Can you work these out from the model? Positions are in its coordinate system, mm. A direction names the side the tool comes from. Round coordinates to 2 decimals unless told otherwise and drop trailing zeros. Loops run counter-clockwise (first coordinate to the right, second up) from the corner with the lowest first, then second, coordinate; pieces in that order, holes last.
from build123d import *

# Parameters (mm, degrees)
BOSS_EXTRUDE1_DEPTH = 150
SKETCH2_R           = 35
SKETCH2_R_2         = 32.5
BOSS_EXTRUDE2_DEPTH = 14
SKETCH3_R           = 9
BOSS_EXTRUDE3_DEPTH = 8
SKETCH5_R           = 3.4
CUT_EXTRUDE1_DEPTH  = 14
CUT_EXTRUDE4_DEPTH  = 154
CUT_EXTRUDE6_START  = -4
CUT_EXTRUDE6_DEPTH  = 4
CUT_EXTRUDE7_START  = -4
CUT_EXTRUDE7_DEPTH  = 4
SKETCH13_R          = 3.4
CUT_EXTRUDE8_DEPTH  = 10
CIRPATTERN1_COUNT   = 3


with BuildPart() as part:
    # Sketch1 → Boss-Extrude1 (new body)
    with BuildSketch(Plane.YZ):
        Polygon((-60, -45), (-60, 45), (60, 45), (60, -45), (56, -45), (56, 41), (-56, 41), (-56, -45), align=None)
    extrude(amount=BOSS_EXTRUDE1_DEPTH)

    # Sketch2 → Boss-Extrude2 (add)
    with BuildSketch(Plane(origin=(0, 60, 0), x_dir=(-1, 0, 0), z_dir=(0, 1, 0))):
        with Locations(Location((-105.539679059, 0.129309752, 0), (0, 0, 270))):
            Circle(SKETCH2_R)
        with Locations(Location((-105.539679059, 0.129309752, 0), (0, 0, 90))):
            Circle(SKETCH2_R_2, mode=Mode.SUBTRACT)
    extrude(amount=BOSS_EXTRUDE2_DEPTH)

    # Sketch3 → Boss-Extrude3 (add)
    with BuildSketch(Plane(origin=(0, 60, 0), x_dir=(-1, 0, 0), z_dir=(0, 1, 0))):
        with Locations(Location((-105.539679059, 0.129309752, 0), (0, 0, 270))):
            Circle(SKETCH3_R)
        with BuildLine():
            Line((-109.989679059, -5.274161354), (-101.089679059, -5.274161354))
            ThreePointArc((-101.089679059, -5.274161354), (-105.539679059, 7.129309752), (-109.989679059, -5.274161354))
        make_face(mode=Mode.SUBTRACT)
    extrude(amount=BOSS_EXTRUDE3_DEPTH)

    # Sketch5 → Cut-Extrude1 (cut)
    with BuildSketch(Plane(origin=(0, 60, 0), x_dir=(-1, 0, 0), z_dir=(0, 1, 0))):
        with Locations(Location((-105.539679059, 0.129309752, 0), (0, 0, 90))):
            Circle(SKETCH5_R)
    extrude(amount=-CUT_EXTRUDE1_DEPTH, mode=Mode.SUBTRACT)

    # Sketch8 → Cut-Extrude4 (cut)
    with BuildSketch(Plane.YZ.offset(150)):
        Polygon((60, 35.129309752), (56, 35.129309752), (56, -34.870690248), (60, -34.870690248), (60, -45), (56, -45), (-60, -45), (-60, 45), (56, 45), (60, 45), align=None)
    extrude(amount=-CUT_EXTRUDE4_DEPTH, mode=Mode.SUBTRACT)

    # Sketch11 → Cut-Extrude6 (cut)
    with BuildSketch(Plane(origin=(0, 60, 0), x_dir=(-1, 0, 0), z_dir=(0, 1, 0)).offset(CUT_EXTRUDE6_START)):
        with BuildLine():
            Line((-150, 35.129309752), (-105.539679059, 35.129309752))
            ThreePointArc((-105.539679059, 35.129309752), (-140.539679059, 0.129309752), (-105.539679059, -34.870690248))
            Line((-105.539679059, -34.870690248), (-150, -34.870690248))
            Line((-150, -34.870690248), (-150, 35.129309752))
        make_face()
    extrude(amount=CUT_EXTRUDE6_DEPTH, mode=Mode.SUBTRACT)

    # Sketch12 → Cut-Extrude7 (cut)
    with BuildSketch(Plane(origin=(0, 60, 0), x_dir=(-1, 0, 0), z_dir=(0, 1, 0)).offset(CUT_EXTRUDE7_START)):
        with BuildLine():
            Line((-105.539679059, 35.129309752), (0, 35.129309752))
            Line((0, 35.129309752), (0, -34.870690248))
            Line((0, -34.870690248), (-105.539679059, -34.870690248))
            ThreePointArc((-105.539679059, -34.870690248), (-70.539679059, 0.129309752), (-105.539679059, 35.129309752))
        make_face()
    extrude(amount=CUT_EXTRUDE7_DEPTH, mode=Mode.SUBTRACT)

    # Sketch13 → Cut-Extrude8 (cut)
    with BuildSketch(Plane.XZ.offset(-56)):
        with Locations(Location((105.539679059, 20.129309752, 0), (0, 0, 270))):
            Circle(SKETCH13_R)
    cut_extrude8 = extrude(amount=-CUT_EXTRUDE8_DEPTH, mode=Mode.SUBTRACT)

    # CirPattern1: Cut-Extrude8 ×3 about axis
    cirpattern1_axis = Axis((105.539679059, 0, 0.129309752), (0, 1, 0))
    for i in range(1, CIRPATTERN1_COUNT):
        add(cut_extrude8.rotate(cirpattern1_axis, i * 360 / CIRPATTERN1_COUNT), mode=Mode.SUBTRACT)


solid = part.part
(1) For faces 5 (the cylindrical face through (108.91, 57.97, 20.57)), 6 (the flat face through (105, 60, 4)), which set-ups out of +Z, -Z, +X, -X, +Y, -Y let a thin tool reach every point of the face, with its end or its side?
Worked answers:
face 5: +Y, -Y
face 6: +Y
(2) If we section it at C-C, the plane z = -1.5: List the corners of the cut face in (x, y) for me.
Worked answers:
outline: (70.58, 56) - (102.56, 56) - (102.56, 60) - (98.73, 60) - (98.73, 68) - (96.69, 68) - (96.69, 60) - (73.08, 60) - (73.08, 74) - (70.58, 74) - close; (108.52, 56) - (140.5, 56) - (140.5, 74) - (138, 74) - (138, 60) - (114.39, 60) - (114.39, 68) - (112.35, 68) - (112.35, 60) - (108.52, 60) - close
(3) If we mould it in two halves opening along X, with no side actions, what happens to faces 1 (the cylindrical face through (126.84, 64.87, 27.9)), 2 (the flat face through (113, 56, 0)), 3 (the cylindrical face through (108.91, 58.03, -0.31)), 4 (the cylindrical face through (123.01, 57.972, -6.474))? For each: released by +X, released by -X, zero draft, split by the parting line, or undercut.
Worked answers:
face 1: split by the parting line
face 2: zero draft
face 3: undercut
face 4: undercut
(4) If I drill on line 1 (Y direction, x = 90, z = 17); line 2 (X direction, y = 67.75, z = 1.5); line 3 (Z direction, x = 105, y = 72), over which ranges is the centre line in solid material (lowest first)?
Worked answers:
line 1: y = 56 to 60
line 2: x = 70.57 to 73.07, 96.64 to 98.68, 112.4 to 114.43, 138.01 to 140.51
line 3: z = -34.87 to -32.37, 32.62 to 35.13
(5) If we section it at B-B, the plane x = 103: List the corners of the cut face in (y, z) for me.
Worked answers:
outline: (56, -34.78) - (74, -34.78) - (74, -32.27) - (60, -32.27) - (60, -8.5) - (68, -8.5) - (68, -5.27) - (60, -5.27) - (60, -2.13) - (56, -2.13) - close; (56, 2.39) - (60, 2.39) - (60, 6.65) - (68, 6.65) - (68, 8.76) - (60, 8.76) - (60, 17.87) - (56, 17.87) - close; (56, 22.39) - (60, 22.39) - (60, 32.53) - (74, 32.53) - (74, 35.04) - (56, 35.04) - close
(6) Will these pins go through, and if not, where does the flat tip stop? P1, Ø5.5, axis at x = 105.54, z = 20.13, coming from the +Y side; P2, Ø1, axis at x = 100, y = 60, coming from the -Z side; P3, Ø5, axis at x = 113.5, y = 69.5, coming from the -Z side; P4, Ø4, axis at x = 91, y = 59, coming from the -Z side.
Worked answers:
P1: passes through
P2: stops at z = -34.51
P3: stops at z = -34.44
P4: stops at z = -32.55
(7) If we section it at A-A, the plane y = 62.5: List the corners of the cut face in (x, z) for me.
Worked answers:
outline: circle Ø70 at (105.54, 0.13); circle Ø18 at (105.54, 0.13); hole circle Ø65 at (105.54, 0.13); hole (101.09, -5.27) - (109.99, -5.27) arc R7 ccw (long way) to start
(8) If we section it at D-D, the plane x = 86: List the corners of the cut face in (y, z) for me, then the cut area to 3 significant figures.
Worked answers:
outline: (56, -28.91) - (74, -28.91) - (74, -25.84) - (60, -25.84) - (60, -12.45) - (56, -12.45) - close; (56, -7.29) - (60, -7.29) - (60, 26.1) - (74, 26.1) - (74, 29.17) - (56, 29.17) - close
area: 298 mm2
